CAD build for the part. Positions are in the model's coordinates, mm. Face numbers are marked on the shaded views. A direction names the side the tool comes from. Give positions to 0.01 mm unless a question says otherwise; leave off trailing zeros. Loops run counter-clockwise (first coordinate to the right, second up) from the corner with the lowest first, then second, coordinate; pieces in that order, holes last.
Autodesk Inventor part; units mm, degrees
ref_plane "YZ Plane" through (0, 0, 0) normal (1, 0, 0) x (0, 1, 0)
ref_plane "XZ Plane" through (0, 0, 0) normal (0, 1, 0) x (-1, 0, 0)
ref_plane "XY Plane" through (0, 0, 0) normal (0, 0, 1) x (1, 0, 0)
sketch "Sketch1" plane through (0, 0, 0) normal (1, 0, 0) x (0, 1, 0)
  line L0 (0, 0) -> (51, 0)
  line L1 (51, 0) -> (51, 2)
  line L2 (51, 2) -> (0, 2)
  line L3 (-2, 0) -> (-2, -51)
  line L4 (-2, -51) -> (0, -51)
  line L5 (0, -51) -> (0, 0)
  line L6 (0, 0) -> (-2, 0)
  line L7 (-2, 0) -> (-2, 2)
  line L8 (-2, 2) -> (0, 2)
  line L9 (0, 2) -> (0, 0)
  dimension "d0" = 51
  dimension "d1" = 2
  dimension "d2" = 2
  dimension "d3" = 51
extrude "Extrusion1" add sketch "Sketch1" along normal blind 50
sketch "Sketch2" plane through (0, 0, 0) normal (0, 0, -1) x (-1, 0, 0)
  line L0 (0, 51) -> (-50, 51)
  line L1 (-25, 51) -> (-25, 30)
  circle A0 centre (-25, 30) radius 11
  line L2 (-25, 51) -> (-9.5, 51)
  line L3 (-25, 30) -> (-9.5, 30)
  line L4 (-9.5, 30) -> (-9.5, 45.5)
  line L5 (-9.5, 30) -> (-9.5, 14.5)
  circle A1 centre (-9.5, 14.5) radius 2
  circle A2 centre (-9.5, 45.5) radius 2
  circle A3 centre (-40.5, 14.5) radius 2
  circle A4 centre (-40.5, 45.5) radius 2
  point P0 (0, 0)
  dimension "d6" = 21
  dimension "d7" = 22
  dimension "d8" = 15.5
  dimension "d9" = 15.5
  dimension "d10" = 15.5
  dimension "d11" = 4
  dimension "d12" = 4
extrude "Extrusion2" cut sketch "Sketch2" against normal blind 50
sketch "Sketch3" plane through (0, 0, 0) normal (0, 1, 0) x (1, 0, 0)
  line L0 (0, 51) -> (50, 51)
  line L1 (25, 51) -> (25, 36)
  line L2 (25, 36) -> (25, 13)
  circle A0 centre (25, 13) radius 3
  circle A1 centre (25, 36) radius 3
  point P0 (0, 0)
  dimension "d15" = 15
  dimension "d16" = 23
  dimension "d17" = 6
  dimension "d18" = 6
extrude "Extrusion3" cut sketch "Sketch3" against normal blind 50
sketch "Sketch4" plane through (50, 0, 0) normal (1, 0, 0) x (0, 0, -1)
  line L0 (-2, 51) -> (-2, -2)
  line L1 (-2, -2) -> (51, -2)
  line L2 (51, -2) -> (51, 51)
  line L3 (51, 51) -> (-2, 51)
  line L4 (-2, 51) -> (-2, -2)
  line L5 (-2, 51) -> (51, -2)
  point P0 (0, 0)
  dimension "d21" = 53
extrude "Extrusion4" add sketch "Sketch4" along normal blind 2 contours L5 L1 L0
sketch "Sketch5" plane through (0, 0, 0) normal (-1, 0, 0) x (0, 0, 1)
  line L0 (2, -2) -> (-51, -2)
  line L1 (2, -2) -> (-51, -2)
  line L2 (-51, -2) -> (-51, 51)
  line L3 (-51, 51) -> (2, 51)
  line L4 (2, 51) -> (2, -2)
  line L5 (-51, -2) -> (2, 51)
  point P0 (0, 0)
  dimension "d24" = 53
  dimension "d25" = 53
extrude "Extrusion5" add sketch "Sketch5" along normal blind 2 contours L0 L5 L4
properties part number "NEMA17-3030-m6-holder" material "Aluminum 6061"
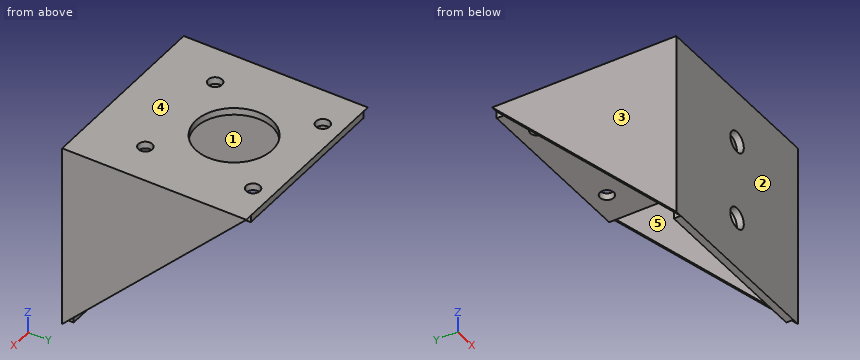
1. Saw through at C-C, the plane z = -13. List the corners of the cut face in (x, y).
Responses:
outline: (-2, -2) - (22, -2) - (22, 0) - (0, 0) - (0, 36) - (-2, 36) - close; (28, -2) - (52, -2) - (52, 36) - (50, 36) - (50, 0) - (28, 0) - close
2. Drop flat-ended pins along their axis: pin 1 (15 mm diameter, centred on x = 12.5, z = -15, fed in from +Y); pin 2 (2 mm diameter, centred on x = 24, y = 14, fed in from -Z). Give the stop position or say it passes through.
Responses:
pin 1: stops at y = 0
pin 2: stops at z = 0
3. Probe line 1 along Z through (x, y) = (25, -1.25); line 2 along X through (y, z) = (30, 1.2); line 3 along X through (y, z) = (28.5, -9.5). List the from-to ranges inside material, lowest first.
Responses:
line 1: z = -51 to -39, -33 to -16, -10 to 2
line 2: x = -2 to 14, 36 to 52
line 3: x = -2 to 0, 50 to 52
4. Saw through at D-D, the plane y = 45.5. List the corners of the cut face in (x, z), and give its area (3 significant figures).
Responses:
outline: (-2, -3.5) - (0, -3.5) - (0, 0) - (7.5, 0) - (7.5, 2) - (-2, 2) - close; (11.5, 0) - (38.5, 0) - (38.5, 2) - (11.5, 2) - close; (42.5, 0) - (50, 0) - (50, -3.5) - (52, -3.5) - (52, 2) - (42.5, 2) - close
area: 106 mm2
5. Tool access for the marked faces 4 and 5: list every direction of +Z, -Z, +X, -X, +Y, -Y with a clear straight run to the whole face (end or side of a thin tool).
Responses:
face 4: +Z, +X, -X, +Y, -Y
face 5: -Z, +Y
6. Saw through at A-A, the plane x = 25. List the corners of the cut face in (y, z), and give its area (3 significant figures).
Responses:
outline: (-2, -51) - (0, -51) - (0, -39) - (-2, -39) - close; (-2, -33) - (0, -33) - (0, -16) - (-2, -16) - close; (-2, -10) - (0, -10) - (0, 0) - (19, 0) - (19, 2) - (-2, 2) - close; (41, 0) - (51, 0) - (51, 2) - (41, 2) - close
area: 140 mm2
7. Pull direction X, two halves, no side cores. Call the marked faces 1, 2 and 3: released by +X, released by -X, zero draft, split by the parting line, or undercut.
Responses:
face 1: undercut
face 2: zero draft
face 3: released by -X
8. Saw through at B-B, the plane y = 30. List the corners of the cut face in (x, z), and give its area (3 significant figures).
Responses:
outline: (-2, -19) - (0, -19) - (0, 0) - (14, 0) - (14, 2) - (-2, 2) - close; (36, 0) - (50, 0) - (50, -19) - (52, -19) - (52, 2) - (36, 2) - close
area: 140 mm2
